Check sheet for the drawn part. Datum: minimum x, y, z corner. Units: mm. A direction names the side the tool comes from. Coordinates: 2 decimals unless noted, no trailing zeros. Loops run counter-clockwise (first coordinate to the right, second up) from the corner with the lowest first, then second, coordinate; pieces in that order, holes last.
Q1. Go/stop test with flat-tipped pins: P1, Ø4, axis at x = 8.5, z = 6.5, coming from the -Y side; P2, Ø2, axis at x = 11.11, y = 5.15, coming from the +Z side; P3, Ø4, axis at y = 3.5, z = 4, coming from the +X side; P4, Ø1.9, axis at y = 4.5, z = 16, coming from the -X side. Record where each tip stops, or that it passes through.
Q2. Mould release check, pull along X, two halves, no side actions. Record for the marked faces 6, 7, 8 and 9: +X half, -X half, draft (parallel to the pull), parting line (faces both ways), or undercut.
Q3. Sectioned sample at B-B (x = 11.11). Enter the section's corners in (y, z), then the cut area to 3 significant figures.
Q4. Access from +Z, -Z, +X, -X, +Y, -Y to the whole of each face (thin tool, end or side, straight path). Record for the marked faces 1, 2, 3, 4 and 5.
Q5. Sectioned sample at C-C (z = 20). Enter the section's corners in (x, y).
Q6. Sectioned sample at A-A (y = 5.15). Enter the section's corners in (x, z), then the cut area to 3 significant figures.
Q7. Material ranges on probe 1 along Y at (x, z) = (11.11, 7.9); probe 2 along X at (y, z) = (7.25, 16.5); probe 3 along Z at (x, y) = (12, 7), recorded low to high.
Q8. Sectioned sample at D-D (y = 9.5). Enter the section's corners in (x, z), then the cut area to 3 significant figures.
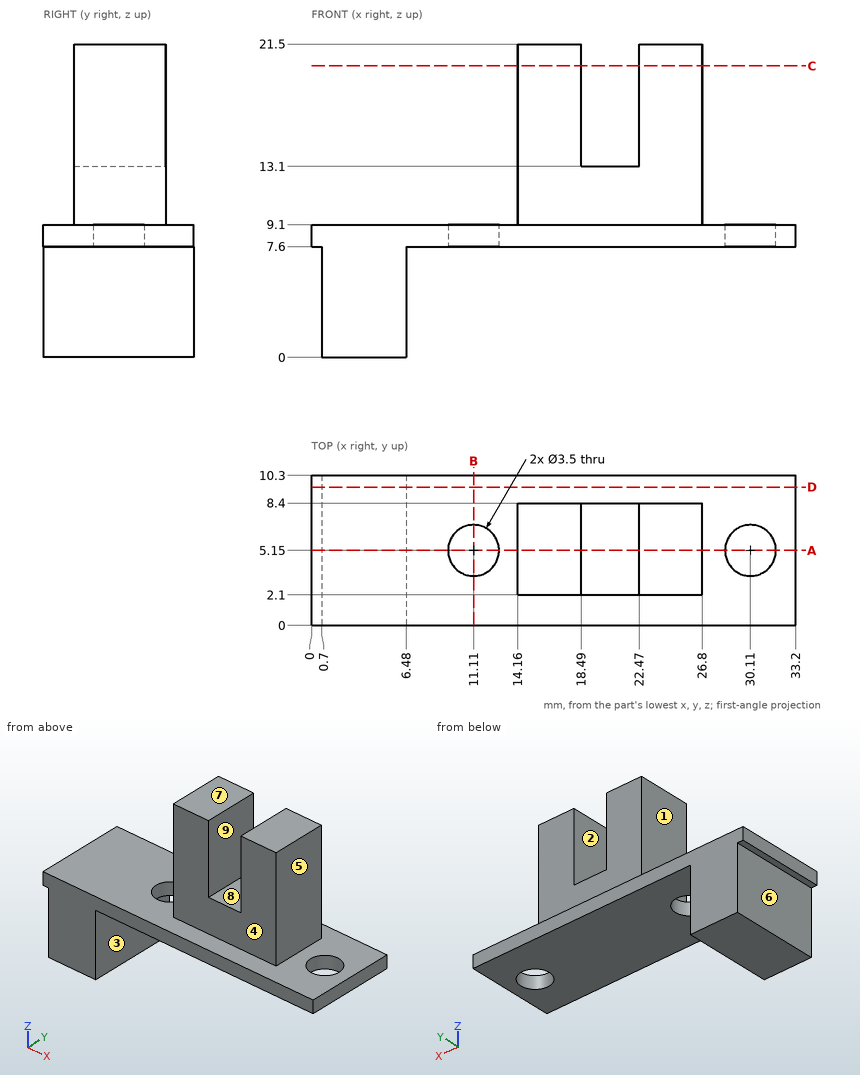
Geometry check:
1. P1: stops at y = 0
1. P2: passes through
1. P3: stops at x = 6.48
1. P4: stops at x = 14.16
2. face 6: -X half
2. face 7: draft
2. face 8: undercut
2. face 9: undercut
3. outline: (0, 7.6) - (3.4, 7.6) - (3.4, 9.1) - (0, 9.1) - close; (6.9, 7.6) - (10.3, 7.6) - (10.3, 9.1) - (6.9, 9.1) - close
3. area: 10.2 mm2
4. face 1: +Z, -X, +Y, -Y
4. face 2: +Z, +Y, -Y
4. face 3: -Z, +X, +Y, -Y
4. face 4: +Z, +X, -X, -Y
4. face 5: +Z, +X, +Y, -Y
5. outline: (14.16, 2.1) - (18.49, 2.1) - (18.49, 8.4) - (14.16, 8.4) - close; (22.47, 2.1) - (26.8, 2.1) - (26.8, 8.4) - (22.47, 8.4) - close
6. outline: (0, 7.6) - (0.7, 7.6) - (0.7, 0) - (6.48, 0) - (6.48, 7.6) - (9.36, 7.6) - (9.36, 9.1) - (0, 9.1) - close; (12.86, 7.6) - (28.36, 7.6) - (28.36, 9.1) - (26.8, 9.1) - (26.8, 21.5) - (22.47, 21.5) - (22.47, 13.1) - (18.49, 13.1) - (18.49, 21.5) - (14.16, 21.5) - (14.16, 9.1) - (12.86, 9.1) - close; (31.86, 7.6) - (33.2, 7.6) - (33.2, 9.1) - (31.86, 9.1) - close
6. area: 207 mm2
7. probe 1: y = 0 to 3.4, 6.9 to 10.3
7. probe 2: x = 14.16 to 18.49, 22.47 to 26.8
7. probe 3: z = 7.6 to 9.1
8. outline: (0, 7.6) - (0.7, 7.6) - (0.7, 0) - (6.48, 0) - (6.48, 7.6) - (33.2, 7.6) - (33.2, 9.1) - (0, 9.1) - close
8. area: 93.7 mm2
